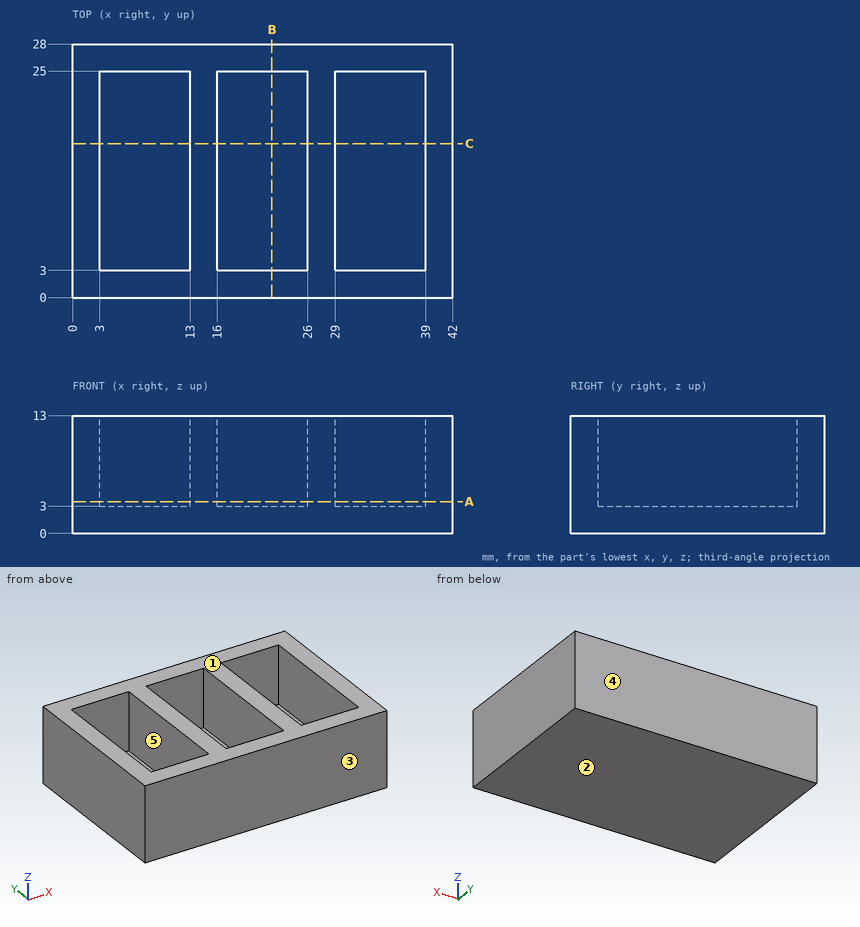
Here's the drawing with two shaded views (mm, measured from the low corner). I have some questions. A direction names the side the tool comes from. Round coordinates to 2 decimals unless told otherwise and drop trailing zeros. Write each loop counter-clockwise with the first axis right and the second up, starting at its lowest first coordinate (ties: lowest second). Pieces come first, ordered by that corner, then holes. Notation, with made-up numbers: M 70.25,14.25 L 95.25,14.25 A22 ccw 95.25,40.25 Z; hole C 14.5,89.25 d5. An arc over 180 degrees is marked long. Answer in a Markdown table with one row per item. Add a question column.
Q1. Imagine slicing it at B-B (x = 22). Please give me the cut outline in (y, z), then the cut area to 3 significant figures.
Q2. Imagine slicing it at C-C (y = 17). Please give me the cut outline in (x, z), then the cut area to 3 significant figures.
Q3. If we mould it in two halves opening along Z, with no side actions, what happens to the marked faces 1, 2 and 3? For each: +Z half, -Z half, draft (parallel to the pull), parting line (faces both ways), or undercut.
Q4. Imagine slicing it at A-A (z = 3.5). Please give me the cut outline in (x, y).
Q5. On a 3-axis mill with a long thin cutter (end or side, diameter ignored), from which of +Z, -Z, +X, -X, +Y, -Y can I reach the whole of each face in a straight line? I mean the marked faces 4 and 5. Say none if no direction works.
Q6. If I drill on line 1 (X direction, y = 13.25, z = 7.5); line 2 (Y direction, x = 37, z = 4); line 3 (Z direction, x = 23, y = 8.5), over which ranges is the centre line in solid material (lowest first)? Write a range as from..to.
Q7. Will this pin go through, and if not, where does the flat tip stop? pin 1 Ø5 at (x, y) = (33.5, 9) entering from +Z.
Values:
| question | item | result |
|---|---|---|
| 1 | outline | M 0,0 L 28,0 L 28,13 L 25,13 L 25,3 L 3,3 L 3,13 L 0,13 Z |
| 1 | area | 144 mm^2 |
| 2 | outline | M 0,0 L 42,0 L 42,13 L 39,13 L 39,3 L 29,3 L 29,13 L 26,13 L 26,3 L 16,3 L 16,13 L 13,13 L 13,3 L 3,3 L 3,13 L 0,13 Z |
| 2 | area | 246 mm^2 |
| 3 | face 1 | +Z half |
| 3 | face 2 | -Z half |
| 3 | face 3 | draft |
| 4 | outline | M 0,0 L 42,0 L 42,28 L 0,28 Z; hole M 3,3 L 13,3 L 13,25 L 3,25 Z; hole M 16,3 L 26,3 L 26,25 L 16,25 Z; hole M 29,3 L 39,3 L 39,25 L 29,25 Z |
| 5 | face 4 | +Z, -Z, +X, -X, +Y |
| 5 | face 5 | +Z |
| 6 | line 1 | 0..3, 13..16, 26..29, 39..42 |
| 6 | line 2 | 0..3, 25..28 |
| 6 | line 3 | 0..3 |
| 7 | pin 1 | z = 3 |
